```python
from build123d import *

# Parameters (mm, degrees)
SKETCH1_W           = 155.7
SKETCH1_H           = 35.6
BOSS_EXTRUDE1_DEPTH = 14
SKETCH3_R           = 1.85
CUT_EXTRUDE1_DEPTH  = 82.076892516
SKETCH4_W           = 20
SKETCH4_H           = 11
CUT_EXTRUDE2_DEPTH  = 158.338266166
CUT_EXTRUDE3_DEPTH  = 87.740892894


with BuildPart() as part:
    # Sketch1 → Boss-Extrude1 (new body)
    with BuildSketch(Plane(origin=(0, 0, 0), x_dir=(1, 0, 0), z_dir=(0, 1, 0))):
        Rectangle(SKETCH1_W, SKETCH1_H)
    extrude(amount=BOSS_EXTRUDE1_DEPTH)

    # Sketch3 → Cut-Extrude1 (cut, through all)
    with BuildSketch(Plane(origin=(0, 14, 0), x_dir=(1, 0, 0), z_dir=(0, 1, 0))):
        with Locations(Location((-71.4375, 0, 0), (0, 0, 270))):
            Circle(SKETCH3_R)
        with Locations(Location((-55.5575, 0, 0), (0, 0, 270))):
            Circle(SKETCH3_R)
        with Locations(Location((-39.6775, 0, 0), (0, 0, 270))):
            Circle(SKETCH3_R)
        with Locations(Location((-23.7975, 0, 0), (0, 0, 270))):
            Circle(SKETCH3_R)
        with Locations(Location((-7.9175, 0, 0), (0, 0, 270))):
            Circle(SKETCH3_R)
        with Locations(Location((7.9625, 0, 0), (0, 0, 270))):
            Circle(SKETCH3_R)
        with Locations(Location((23.8425, 0, 0), (0, 0, 270))):
            Circle(SKETCH3_R)
        with Locations(Location((39.7225, 0, 0), (0, 0, 270))):
            Circle(SKETCH3_R)
        with Locations(Location((55.6025, 0, 0), (0, 0, 270))):
            Circle(SKETCH3_R)
        with Locations(Location((71.4825, 0, 0), (0, 0, 270))):
            Circle(SKETCH3_R)
    extrude(amount=-CUT_EXTRUDE1_DEPTH, mode=Mode.SUBTRACT)

    # Sketch4 → Cut-Extrude2 (cut, through all)
    with BuildSketch(Plane.ZY.offset(77.85)):
        with Locations((0, 8.5)):
            Rectangle(SKETCH4_W, SKETCH4_H)
    extrude(amount=-CUT_EXTRUDE2_DEPTH, mode=Mode.SUBTRACT)

    # Sketch5 → Cut-Extrude3 (cut, through all)
    with BuildSketch(Plane.XY.offset(17.8)):
        with BuildLine():
            Line((-74.71, 9), (-74.71, 15))
            Line((-74.71, 15), (-68.21, 15))
            Line((-68.21, 15), (-68.21, 9))
            ThreePointArc((-68.21, 9), (-71.46, 5.75), (-74.71, 9))
        make_face()
        with BuildLine():
            Line((-52.33, 15), (-52.33, 9))
            ThreePointArc((-52.33, 9), (-55.58, 5.75), (-58.83, 9))
            Line((-58.83, 9), (-58.83, 15))
            Line((-58.83, 15), (-52.33, 15))
        make_face()
        with BuildLine():
            Line((-36.45, 15), (-36.45, 9))
            ThreePointArc((-36.45, 9), (-39.7, 5.75), (-42.95, 9))
            Line((-42.95, 9), (-42.95, 15))
            Line((-42.95, 15), (-36.45, 15))
        make_face()
        with BuildLine():
            Line((-20.57, 15), (-20.57, 9))
            ThreePointArc((-20.57, 9), (-23.82, 5.75), (-27.07, 9))
            Line((-27.07, 9), (-27.07, 15))
            Line((-27.07, 15), (-20.57, 15))
        make_face()
        with BuildLine():
            Line((-4.69, 15), (-4.69, 9))
            ThreePointArc((-4.69, 9), (-7.94, 5.75), (-11.19, 9))
            Line((-11.19, 9), (-11.19, 15))
            Line((-11.19, 15), (-4.69, 15))
        make_face()
        with BuildLine():
            Line((11.19, 15), (11.19, 9))
            ThreePointArc((11.19, 9), (7.94, 5.75), (4.69, 9))
            Line((4.69, 9), (4.69, 15))
            Line((4.69, 15), (11.19, 15))
        make_face()
        with BuildLine():
            Line((27.07, 15), (27.07, 9))
            ThreePointArc((27.07, 9), (23.82, 5.75), (20.57, 9))
            Line((20.57, 9), (20.57, 15))
            Line((20.57, 15), (27.07, 15))
        make_face()
        with BuildLine():
            Line((42.95, 15), (42.95, 9))
            ThreePointArc((42.95, 9), (39.7, 5.75), (36.45, 9))
            Line((36.45, 9), (36.45, 15))
            Line((36.45, 15), (42.95, 15))
        make_face()
        with BuildLine():
            Line((58.83, 15), (58.83, 9))
            ThreePointArc((58.83, 9), (55.58, 5.75), (52.33, 9))
            Line((52.33, 9), (52.33, 15))
            Line((52.33, 15), (58.83, 15))
        make_face()
        with BuildLine():
            Line((74.71, 15), (74.71, 9))
            ThreePointArc((74.71, 9), (71.46, 5.75), (68.21, 9))
            Line((68.21, 9), (68.21, 15))
            Line((68.21, 15), (74.71, 15))
        make_face()
    extrude(amount=-CUT_EXTRUDE3_DEPTH, mode=Mode.SUBTRACT)


solid = part.part
```
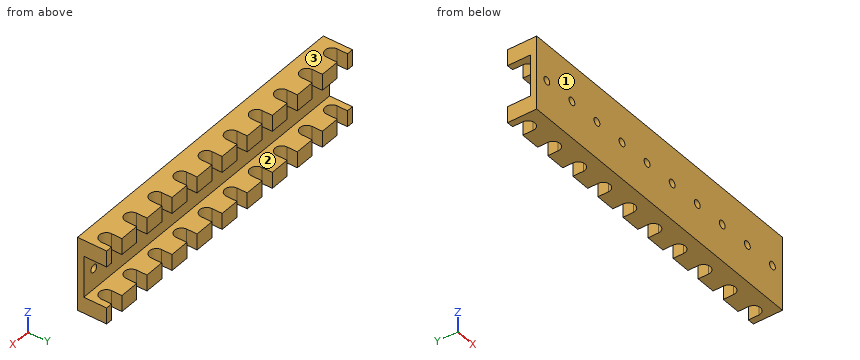
Check sheet for the modelled part. Datum: model origin and axes. Units: mm. Face numbers are marked on the shaded views. Round coordinates to 2 decimals unless told otherwise and drop trailing zeros. Order: outer loops, then holes, each group sorted by start corner. A loop starts at its lowest first (then second) coordinate and runs counter-clockwise, first axis right, second up. Notation, with made-up numbers: (35.5, -24.5) -> (52.5, -24.5) arc R27 cw to (52.5, -6.5) -> close; hole circle Ø11 at (63.25, 61). An arc over 180 degrees is marked (long way). One line per item, written item: value. Start each with the question number.
Q1. Gauge pin test, flat ends, axial feed: pin 1 Ø3 at (x, z) = (7.96, 0) entering from -Y; pin 2 Ø1.5 at (x, z) = (-28.5, 1) entering from +Y. Record the tip position at first contact, or that the pin passes through.
Q2. Cross-section at B-B (x = -50). Record the boundary of the cut face in (y, z).
Q3. Cross-section at A-A (y = 1.5). Give the number of separate pieces and of enclosed holes in the cut face, and give its area (3 significant figures).
Q4. Mould release check, pull along Z, two halves, no side actions. Record for the marked faces 1, 2 and 3: pulls with the +Z half, pulls with the -Z half, needs draft (parallel to the pull), parting line crosses it, or undercut.
Q5. Thickness scan on line 1 (Z direction, x = 18.5, y = 10.25); line 2 (Y direction, x = 15, z = 4); line 3 (Z direction, x = 9, y = 2.5). Record the ranges inside material, lowest first.
Completed:
1. pin 1: passes through
1. pin 2: stops at y = 3
2. outline: (0, -17.8) -> (14, -17.8) -> (14, -10) -> (3, -10) -> (3, 10) -> (14, 10) -> (14, 17.8) -> (0, 17.8) -> close
3. separate pieces: 1
3. enclosed holes: 10
3. area: 5,440 mm²
4. face 1: needs draft
4. face 2: undercut
4. face 3: pulls with the +Z half
5. line 1: z = -17.8 to -10, 10 to 17.8
5. line 2: y = 0 to 3
5. line 3: z = -17.8 to -1.53, 1.53 to 17.8
